Source: CAD feature listing. Evaluate the final solid. Frame: model axes, mm. Face numbers are marked on the shaded views. Give positions to 0.01 mm unless a question says otherwise; leave off trailing zeros. Order: outer loops, then holes, each group sorted by start corner. A loop starts at its lowest first (then second) coordinate and runs counter-clockwise, first axis right, second up. Notation, with made-up numbers: (-21, 17.5) -> (28, 17.5) arc R32 cw to (28, 49.5) -> close; hole circle Ø8 at (2.5, 0). An arc over 180 degrees is marked (long way). Use CSV: the item, a comma, the result in double quotes.
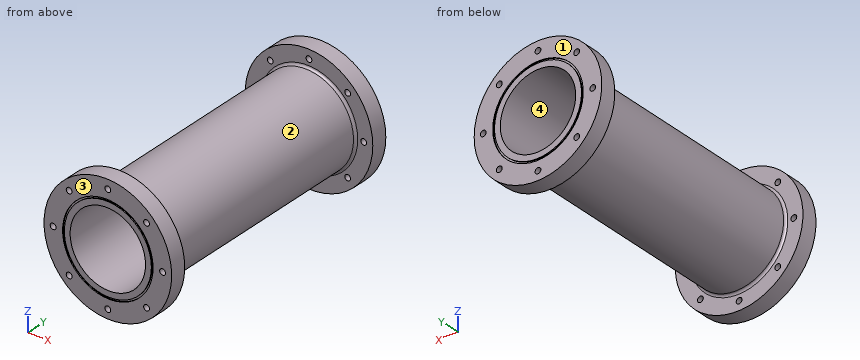
```python
from build123d import *

# Parameters (mm, degrees)
SKETCH2_R               = 50.8
SKETCH2_R_2             = 41.275
BASE_CYLINDER_DEPTH     = 292.1
SKETCH3_R               = 69.85
SKETCH3_R_2             = 41.275
AFT_FLANGE_DEPTH        = 17.78
SKETCH4_R               = 69.85
SKETCH4_R_2             = 41.275
FORWARD_FLANGE_DEPTH    = 17.78
SKETCH6_R               = 49.53
SKETCH6_R_2             = 47.625
O_RING_SLOT_1_DEPTH     = 1.1176
SKETCH7_R               = 49.53
SKETCH7_R_2             = 47.625
O_RING_SLOT_2_DEPTH     = 1.1176
SKETCH8_R               = 3.175
CUT_EXTRUDE4_DEPTH      = 1
CUT_EXTRUDE4_DEPTH_BACK = 293.1
FILLET1_R               = 2.54


with BuildPart() as part:
    # Sketch2 → Base Cylinder (new body)
    with BuildSketch(Plane(origin=(0, 0, 0), x_dir=(1, 0, 0), z_dir=(0, 1, 0))):
        Circle(SKETCH2_R)
        Circle(SKETCH2_R_2, mode=Mode.SUBTRACT)
    extrude(amount=BASE_CYLINDER_DEPTH)

    # Sketch3 → Aft Flange (add)
    with BuildSketch(Plane.XZ):
        Circle(SKETCH3_R)
        Circle(SKETCH3_R_2, mode=Mode.SUBTRACT)
    extrude(amount=-AFT_FLANGE_DEPTH)

    # Sketch4 → Forward Flange (add)
    with BuildSketch(Plane(origin=(0, 292.1, 0), x_dir=(1, 0, 0), z_dir=(0, 1, 0))):
        Circle(SKETCH4_R)
        Circle(SKETCH4_R_2, mode=Mode.SUBTRACT)
    extrude(amount=-FORWARD_FLANGE_DEPTH)

    # Sketch6 → O-Ring Slot 1 (cut)
    with BuildSketch(Plane.XZ):
        Circle(SKETCH6_R)
        Circle(SKETCH6_R_2, mode=Mode.SUBTRACT)
    extrude(amount=-O_RING_SLOT_1_DEPTH, mode=Mode.SUBTRACT)

    # Sketch7 → O-Ring Slot 2 (cut)
    with BuildSketch(Plane(origin=(0, 292.1, 0), x_dir=(1, 0, 0), z_dir=(0, 1, 0))):
        Circle(SKETCH7_R)
        Circle(SKETCH7_R_2, mode=Mode.SUBTRACT)
    extrude(amount=-O_RING_SLOT_2_DEPTH, mode=Mode.SUBTRACT)

    # Sketch8 → Cut-Extrude4 (cut, two sides)
    with BuildSketch(Plane.XZ) as cut_extrude4_sk:
        with Locations((-59.9186, 0)):
            Circle(SKETCH8_R)
        with Locations((-42.368848379, 42.368848379)):
            Circle(SKETCH8_R)
        with Locations((0, 59.9186)):
            Circle(SKETCH8_R)
        with Locations((42.368848379, 42.368848379)):
            Circle(SKETCH8_R)
        with Locations((59.9186, 0)):
            Circle(SKETCH8_R)
        with Locations((42.368848379, -42.368848379)):
            Circle(SKETCH8_R)
        with Locations((0, -59.9186)):
            Circle(SKETCH8_R)
        with Locations((-42.368848379, -42.368848379)):
            Circle(SKETCH8_R)
    extrude(amount=CUT_EXTRUDE4_DEPTH, mode=Mode.SUBTRACT)
    extrude(cut_extrude4_sk.sketch, amount=-CUT_EXTRUDE4_DEPTH_BACK, mode=Mode.SUBTRACT)

    # Fillet1
    fillet1_edges = [part.edges().sort_by_distance(p)[0] for p in [
        (-50.8, 17.78, 0),
        (-50.8, 274.32, 0),
    ]]
    fillet(fillet1_edges, radius=FILLET1_R)


solid = part.part
```
1. Ray query, line 1 along Z through (x, y) = (0, 11) (3 decimals); line 2 along Z through (x, y) = (0, 291.25) (3 decimals); line 3 along Y through (x, z) = (53.5, 32). Return the intervals inside material, ascending.
Answer below:
line 1,"z = -69.85 to -63.094, -56.744 to -41.275, 41.275 to 56.744, 63.094 to 69.85"
line 2,"z = -69.85 to -63.094, -56.744 to -49.53, -47.625 to -41.275, 41.275 to 47.625, 49.53 to 56.744, 63.094 to 69.85"
line 3,"y = 0 to 17.78, 274.32 to 292.1"
2. Mould query, pull axis Y, two halves, no side actions, for the marked faces 1, 2, 3 and 4. Classes: released by +Y, released by -Y, zero draft, split by the parting line, or undercut.
Answer below:
face 1,"released by +Y"
face 2,"undercut"
face 3,"released by -Y"
face 4,"zero draft"
3. Pin query (flat end, axial travel): P1, Ø2, axis at y = 180, z = 20, coming from the +X side; P2, Ø2, axis at x = 45, y = 77, coming from the +Z side; P3, Ø12, axis at y = 135.5, z = 1.5, coming from the -X side. Return the tip coordinate at first contact, or that it passes through.
Answer below:
P1,"stops at x = 47.11"
P2,"stops at z = 25.39"
P3,"stops at x = -50.8"
4. Section query A-A on y = 62.5. Return loops of the section in (x, z) (3 decimals), plus the area to 3 significant figures.
Answer below:
outline,"circle Ø101.6 at (0, 0); hole circle Ø82.55 at (0, 0)"
area,"2,760 mm²"
5. Section query B-B on z = 0. Count the separate pieces of the cut face and the enclosed holes in it, plus the area to 3 significant figures.
Answer below:
separate pieces,"6"
enclosed holes,"0"
area,"6,460 mm²"
